Geometry: final body of the model. Coordinates: model frame, mm. A direction names the side the tool comes from. Give positions to 0.01 mm unless a question says otherwise; leave off trailing zeros. Write each loop counter-clockwise with the first axis right and the second up, starting at its lowest first coordinate (ties: lowest second). Pieces come first, ordered by that corner, then holes. Notation, with made-up numbers: (29.25, 25) -> (81.25, 25) arc R19 ccw to (81.25, 48) -> close; hole circle Ø6 at (58.25, -30.75). An arc over 180 degrees is marked (long way). Use CSV: the item, a comma, the result in double quotes. Start each with the question number.
1) Section C-C (y = -191.5). Output: boundary loops of the cut face in (x, z), plus the area to 3 significant figures.
2) Draft query along Z for faces 1 (the face through (23.846, -237.48, 7.509)), 2 (the face through (-3.441, -385.49, -15.497)). Return one class per face: pulls with the +Z half, pulls with the -Z half, needs draft (parallel to the pull), parting line crosses it, or undercut.
3) Section B-B (z = 10.5). Output: boundary loops of the cut face in (x, y), plus the area to 3 significant figures.
4) Section A-A (x = 0). Output: boundary loops of the cut face in (y, z) (3 decimals).
5) Set-up query: faces 3 (the face through (0, -350, 0)), 4 (the face through (-0.3, -420, -16.3)), 5 (the face through (-19.076, -29.58, 6.007)). Return all of +Z, -Z, +X, -X, +Y, -Y with unobstructed straight access to the full face (end or side cutting, diameter ignored); none if empty.
6) Material intervals for line 1 (Y direction, x = 18.25, z = 0); line 2 (Y direction, x = 21.25, z = 0); line 3 (X direction, y = -143.5, z = 0.5) (3 decimals), sorted ascending. Write a range as [from, to].
7) Contact query for flat-ended pins moving along their axis: P1, Ø5, axis at x = 11.5, z = 4.5, coming from the +Y side; P2, Ø1.5, axis at y = -262, z = 10, coming from the -X side; P3, Ø6, axis at x = 20, y = -265.5, coming from the -Z side; P4, Ø5, axis at y = -30, z = -0.5, coming from the +X side. Output: stop coordinate, or through.
```python
from build123d import *

# Parameters (mm, degrees)
F0_R      = 25
F1_DEPTH  = 420
F2_R      = 15.875
F3_DEPTH  = 70
F4_R      = 3
F4_R_2    = 3.094555
F5_DEPTH  = 48.2
F6_R      = 25
F6_R_2    = 20
F7_DEPTH  = 60
F9_W      = 98.705204
F9_H      = 10
F10_DEPTH = 0.8


with BuildPart() as f1:
    # F0 (on Front) → F1 (new body)
    with BuildSketch(Plane.XZ):
        Circle(F0_R)
    extrude(amount=F1_DEPTH)

    # F2 (on face) → F3 (cut)
    with BuildSketch(Plane.XZ.offset(420)):
        Circle(F2_R)
    extrude(amount=-F3_DEPTH, mode=Mode.SUBTRACT)

    # F4 (on Right) → F5 (cut)
    with BuildSketch(Plane.YZ):
        with Locations((-390, 0)):
            Circle(F4_R)
        with Locations((-368, 0)):
            Circle(F4_R_2)
    extrude(amount=F5_DEPTH, mode=Mode.SUBTRACT)

    # F6 (on face) → F7 (cut)
    with BuildSketch(Plane(origin=(0, 0, 0), x_dir=(-1, 0, 0), z_dir=(0, 1, 0))):
        Circle(F6_R)
        Circle(F6_R_2, mode=Mode.SUBTRACT)
    extrude(amount=-F7_DEPTH, mode=Mode.SUBTRACT)

    # F9 (on offset) → F10 (cut)
    with BuildSketch(Plane.YZ.offset(20)):
        Rectangle(F9_W, F9_H)
    extrude(amount=-F10_DEPTH, mode=Mode.SUBTRACT)


solid = f1.part
```
Answers follow:
1,outline,"circle Ø50 at (0, 0)"
1,area,"1,960 mm^2"
2,face 1,"parting line crosses it"
2,face 2,"undercut"
3,outline,"(-22.69, -420) -> (-11.91, -420) -> (-11.91, -350) -> (11.91, -350) -> (11.91, -420) -> (22.69, -420) -> (22.69, -60) -> (17.02, -60) -> (17.02, 0) -> (-17.02, 0) -> (-17.02, -60) -> (-22.69, -60) -> close"
3,area,"16,700 mm^2"
4,outline,"(-420, -25) -> (-60, -25) -> (-60, -20) -> (0, -20) -> (0, 20) -> (-60, 20) -> (-60, 25) -> (-420, 25) -> (-420, 15.875) -> (-350, 15.875) -> (-350, -15.875) -> (-420, -15.875) -> close"
5,face 3,"-Y"
5,face 4,"+Z, -Z, +X, -X, -Y"
5,face 5,"+Y"
6,line 1,"y = [-420, -393], [-387, -371.09], [-364.91, 0]"
6,line 2,"y = [-420, -393], [-387, -371.09], [-364.91, -60]"
6,line 3,"x = [-24.995, 24.995]"
7,P1,"stops at y = 0"
7,P2,"stops at x = -23.23"
7,P3,"stops at z = -18.33"
7,P4,"stops at x = 19.2"
